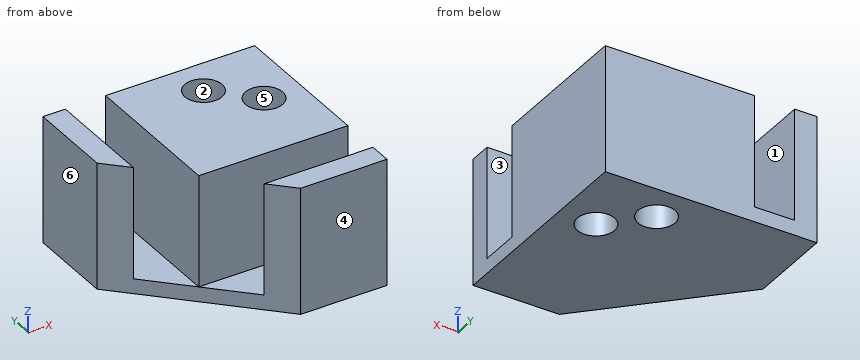
from build123d import *

# Parameters (mm, degrees)
F0_W     = 20
F0_H     = 20
F0_R     = 2.5
F1_DEPTH = 15
F3_DEPTH = 15
F4_R     = 2.5
F5_DEPTH = 2


with BuildPart() as f1:
    # F0 (on Top) → F1 (new body)
    with BuildSketch(Plane.XY):
        with Locations((10, 10)):
            Rectangle(F0_W, F0_H)
        with Locations((15, 10)):
            Circle(F0_R, mode=Mode.SUBTRACT)
        with Locations((10, 15)):
            Circle(F0_R, mode=Mode.SUBTRACT)
    extrude(amount=F1_DEPTH)



with BuildPart() as f3:
    # F2 (on Top) → F3 (new body, through all)
    with BuildSketch(Plane.XY):
        Polygon((-5.4, 8.4), (-5.4, 20), (-8.4, 20), (-8.4, 8.4), (-5.4, 5.4), align=None)
        Polygon((20, -8.4), (20, -5.4), (8.4, -5.4), (5.4, -5.4), (8.4, -8.4), align=None)
    extrude(amount=F3_DEPTH)


with BuildPart() as f1_1:
    add(f1.part)

    add(f3.part)  # F5 merges F3
    # F4 (on face) → F5 (join)
    with BuildSketch(Plane(origin=(0, 0, 0), x_dir=(1, 0, 0), z_dir=(0, 0, -1))):
        Polygon((-8.4, -20), (20, -20), (20, 8.4), (8.4, 8.4), (-8.4, -8.4), align=None)
        with Locations((10, -15)):
            Circle(F4_R, mode=Mode.SUBTRACT)
        with Locations((15, -10)):
            Circle(F4_R, mode=Mode.SUBTRACT)
    extrude(amount=F5_DEPTH)


solid = f1_1.part
Source: CAD feature listing. Evaluate the final solid. Frame: model axes, mm. Face numbers are marked on the shaded views. A direction names the side the tool comes from. Coordinates: 2 decimals unless noted, no trailing zeros. Loops run counter-clockwise (first coordinate to the right, second up) from the corner with the lowest first, then second, coordinate; pieces in that order, holes last. Notation, with made-up numbers: (55.25, -4) - (81.25, -4) arc R16 ccw to (81.25, 11) - close; hole circle Ø8 at (-12, 64.5). An arc over 180 degrees is marked (long way). Return JSON: item names as keys, results as strings.
Q1. Section C-C, the plane y = 10. Return loops of the section in (x, z).
Results:
{"outline": "(-8.4, -2) - (12.5, -2) - (12.5, 15) - (0, 15) - (0, 0) - (-5.4, 0) - (-5.4, 15) - (-8.4, 15) - close; (17.5, -2) - (20, -2) - (20, 15) - (17.5, 15) - close"}
Q2. Section B-B, the plane x = 15. Return loops of the section in (y, z).
Results:
{"outline": "(-8.4, -2) - (7.5, -2) - (7.5, 15) - (0, 15) - (0, 0) - (-5.4, 0) - (-5.4, 15) - (-8.4, 15) - close; (12.5, -2) - (20, -2) - (20, 15) - (12.5, 15) - close"}
Q3. Section A-A, the plane z = 11.25. Return loops of the section in (x, y), plus the area to 3 significant figures.
Results:
{"outline": "(-8.4, 8.4) - (-5.4, 5.4) - (-5.4, 20) - (-8.4, 20) - close; (0, 0) - (20, 0) - (20, 20) - (0, 20) - close; (5.4, -5.4) - (8.4, -8.4) - (20, -8.4) - (20, -5.4) - close; hole circle Ø5 at (10, 15); hole circle Ø5 at (15, 10)", "area": "439 mm2"}
Q4. Material intervals for line 1 along Y through (x, z) = (10, 8.75); line 2 along X through (y, z) = (15, 3.25), sorted ascending.
Results:
{"line 1": "-8.4 to -5.4, 0 to 12.5, 17.5 to 20", "line 2": "-8.4 to -5.4, 0 to 7.5, 12.5 to 20"}
Q5. Access query for the marked faces 1, 2 and 3. Directions: +Z, -Z, +X, -X, +Y, -Y. A direction counts if a zero-diameter tool reaches every point of the face in a straight line with its end or side. Return the directions, or none.
Results:
{"face 1": "+Z, +Y, -Y", "face 2": "+Z, -Z", "face 3": "+Z, +X, -X"}
Q6. Mould query, pull axis Y, two halves, no side actions, for the marked faces 4, 5 and 6. Classes: released by +Y, released by -Y, zero draft, split by the parting line, or undercut.
Results:
{"face 4": "released by -Y", "face 5": "undercut", "face 6": "zero draft"}
Q7. Contact query for flat-ended pins moving along their axis: P1, Ø1, axis at x = -3.5, y = 10.5, coming from the +Z side; P2, Ø10, axis at x = -2.5, y = 11, coming from the +Z side. Output: stop coordinate, or through.
Results:
{"P1": "z = 0", "P2": "z = 15"}
Q8. Section D-D, the plane x = 4.5. Return loops of the section in (y, z).
Results:
{"outline": "(-4.5, -2) - (20, -2) - (20, 15) - (0, 15) - (0, 0) - (-4.5, 0) - close"}
